Design review of the part built by this model. Coordinates are the model's own, in mm. Round coordinates to 2 decimals unless told otherwise and drop trailing zeros. Order: outer loops, then holes, each group sorted by start corner. A loop starts at its lowest first (then second) coordinate and runs counter-clockwise, first axis right, second up. Notation, with made-up numbers: (-2, 17.25) - (14, 17.25) arc R21 ccw to (14, 37.25) - close; hole circle Ø11 at (-3.75, 2.25). An arc over 180 degrees is marked (long way). Use CSV: the item, a comma, the result in double quotes. Start each with the question number.
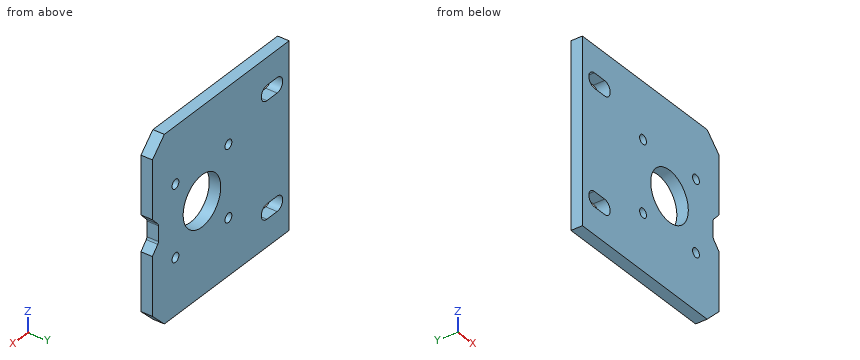
from build123d import *

# Parameters (mm, degrees)
SCHIZZO1_W                   = 80
SCHIZZO1_H                   = 5
ESTRUSIONE_ESTRUSIONE1_DEPTH = 80
SCHIZZO4_R                   = 11
TAGLIO_ESTRUSIONE1_DEPTH     = 6
SCHIZZO6_R                   = 2
TAGLIO_ESTRUSIONE3_DEPTH     = 6
CHAMFER1_SIZE                = 7
CUT_EXTRUDE1_DEPTH           = 6
CUT_EXTRUDE2_DEPTH           = 6
FILLET1_R                    = 1.5
FILLET2_R                    = 1.5


with BuildPart() as part:
    # Schizzo1 → Estrusione-Estrusione1 (new body)
    with BuildSketch(Plane.XY):
        with Locations((40, 2.5)):
            Rectangle(SCHIZZO1_W, SCHIZZO1_H)
    extrude(amount=ESTRUSIONE_ESTRUSIONE1_DEPTH)

    # Schizzo4 → Taglio-Estrusione1 (cut, through all)
    with BuildSketch(Plane(origin=(0, 5, 0), x_dir=(1, 0, 0), z_dir=(0, 1, 0))):
        with Locations((51, -40)):
            Circle(SCHIZZO4_R)
    extrude(amount=-TAGLIO_ESTRUSIONE1_DEPTH, mode=Mode.SUBTRACT)

    # Schizzo6 → Taglio-Estrusione3 (cut, through all)
    with BuildSketch(Plane(origin=(0, 5, 0), x_dir=(1, 0, 0), z_dir=(0, 1, 0))):
        with Locations((35.5, -24.5)):
            Circle(SCHIZZO6_R)
        with Locations((66.5, -24.5)):
            Circle(SCHIZZO6_R)
        with Locations((66.5, -55.5)):
            Circle(SCHIZZO6_R)
        with Locations((35.5, -55.5)):
            Circle(SCHIZZO6_R)
    extrude(amount=-TAGLIO_ESTRUSIONE3_DEPTH, mode=Mode.SUBTRACT)

    # Chamfer1
    chamfer1_edges = [part.edges().sort_by_distance(p)[0] for p in [
        (80, 2.5, 80),
        (80, 2.5, 0),
    ]]
    chamfer(chamfer1_edges, length=CHAMFER1_SIZE)

    # Sketch1 → Cut-Extrude1 (cut, through all)
    with BuildSketch(Plane(origin=(0, 5, 0), x_dir=(1, 0, 0), z_dir=(0, 1, 0))):
        with BuildLine():
            Line((7, -11.75), (13, -11.75))
            ThreePointArc((13, -11.75), (16.25, -15), (13, -18.25))
            Line((13, -18.25), (7, -18.25))
            ThreePointArc((7, -18.25), (3.75, -15), (7, -11.75))
        make_face()
        with BuildLine():
            Line((7, -68.25), (13, -68.25))
            ThreePointArc((13, -68.25), (16.25, -65), (13, -61.75))
            Line((13, -61.75), (7, -61.75))
            ThreePointArc((7, -61.75), (3.75, -65), (7, -68.25))
        make_face()
    extrude(amount=-CUT_EXTRUDE1_DEPTH, mode=Mode.SUBTRACT)

    # Sketch2 → Cut-Extrude2 (cut, through all)
    with BuildSketch(Plane(origin=(0, 5, 0), x_dir=(1, 0, 0), z_dir=(0, 1, 0))):
        Polygon((80, -32.245982949), (76.480308406, -36.096971283), (76.480308406, -43.903028717), (80, -47.754017051), align=None)
    extrude(amount=-CUT_EXTRUDE2_DEPTH, mode=Mode.SUBTRACT)

    # Fillet1
    fillet1_edges = [part.edges().sort_by_distance(p)[0] for p in [
        (76.480308406, 2.5, 36.096971283),
    ]]
    fillet(fillet1_edges, radius=FILLET1_R)

    # Fillet2
    fillet2_edges = [part.edges().sort_by_distance(p)[0] for p in [
        (76.480308406, 2.5, 43.903028717),
    ]]
    fillet(fillet2_edges, radius=FILLET2_R)


solid = part.part
Q1. Take a section at B-B (z = 15). State the section outline as (x, y) points.
Q2. Take a section at A-A (x = 35.5). State the section outline as (y, z) points.
Q3. For L1, parallel to X at y = 2.5, z = 24.5; L2, parallel to Z at x = 51, y = 1.5; L3, parallel to Z at x = 68, y = 4.7, list the stretches that pass through material, from the lowest coordinate up. Write a range as [from, to].
Q4. Take a section at D-D (x = 51). State the section outline as (y, z) points, plus the area to 3 significant figures.
Q5. Take a section at C-C (y = 2.1). State the section outline as (x, z) points, plus the area to 3 significant figures.
Q6. Clearance check with a flat-ended pin moving along its axis: pin 1 (3.5 mm diameter, centred on x = 66.5, z = 55.5, fed in from +Y). State where the tip first meets the part, or that it passes through.
Findings below:
1,outline,"(0, 0) - (3.75, 0) - (3.75, 5) - (0, 5) - close; (16.25, 0) - (80, 0) - (80, 5) - (16.25, 5) - close"
2,outline,"(0, 0) - (5, 0) - (5, 22.5) - (0, 22.5) - close; (0, 26.5) - (5, 26.5) - (5, 53.5) - (0, 53.5) - close; (0, 57.5) - (5, 57.5) - (5, 80) - (0, 80) - close"
3,L1,"x = [0, 33.5], [37.5, 64.5], [68.5, 80]"
3,L2,"z = [0, 29], [51, 80]"
3,L3,"z = [0, 23.18], [25.82, 54.18], [56.82, 80]"
4,outline,"(0, 0) - (5, 0) - (5, 29) - (0, 29) - close; (0, 51) - (5, 51) - (5, 80) - (0, 80) - close"
4,area,"290 mm^2"
5,outline,"(0, 0) - (73, 0) - (80, 7) - (80, 32.25) - (76.87, 35.67) arc R1.5 cw to (76.48, 36.68) - (76.48, 43.32) arc R1.5 cw to (76.87, 44.33) - (80, 47.75) - (80, 73) - (73, 80) - (0, 80) - close; hole (7, 11.75) - (13, 11.75) arc R3.25 ccw to (13, 18.25) - (7, 18.25) arc R3.25 ccw to start; hole (7, 61.75) - (13, 61.75) arc R3.25 ccw to (13, 68.25) - (7, 68.25) arc R3.25 ccw to start; hole circle Ø4 at (35.5, 24.5); hole circle Ø4 at (35.5, 55.5); hole circle Ø22 at (51, 40); hole circle Ø4 at (66.5, 24.5); hole circle Ø4 at (66.5, 55.5)"
5,area,"5,740 mm^2"
6,pin 1,"passes through"
